Here's how the part is built. I have some questions about the finished solid (model axes, mm). Face numbers are marked on the shaded views. A direction names the side the tool comes from. Round coordinates to 2 decimals unless told otherwise and drop trailing zeros. Order: outer loops, then holes, each group sorted by start corner. A loop starts at its lowest first (then second) coordinate and runs counter-clockwise, first axis right, second up. Notation, with made-up numbers: (-29, 45.5) - (11, 45.5) arc R14 ccw to (11, 61.5) - close; hole circle Ø5 at (79.5, -1). An arc over 180 degrees is marked (long way). Answer as a JSON object with one key per item and string values.
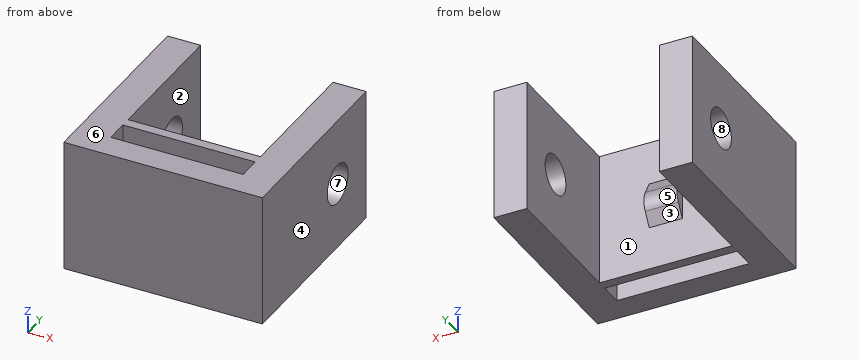
```python
from build123d import *

# Parameters (mm, degrees)
SKETCH1_W           = 10
SKETCH1_H           = 0.75
BOSS_EXTRUDE1_DEPTH = 10
BOSS_EXTRUDE2_DEPTH = 1.25
SKETCH2_5_R         = 1.5
CUT_EXTRUDE1_DEPTH  = 25
FILLET1_R           = 1.5


with BuildPart() as part:
    # Sketch1 → Boss-Extrude1 (new body)
    with BuildSketch(Plane.XY):
        Polygon((-4.83125, 6.8625), (-7.33125, 6.8625), (-7.33125, -8.1375), (7.66875, -8.1375), (7.66875, 6.8625), (5.16875, 6.8625), (5.16875, -3.6375), (5.16875, -4.3875), (5.16875, -6.1375), (-4.83125, -6.1375), (-4.83125, -4.3875), (-4.83125, -3.6375), align=None)
        with Locations((0.16875, -4.0125)):
            Rectangle(SKETCH1_W, SKETCH1_H)
    extrude(amount=BOSS_EXTRUDE1_DEPTH)

    # Sketch2 → Boss-Extrude2 (add, symmetric)
    with BuildSketch(Plane(origin=(0.16875, 0, 0), x_dir=(0, 0, -1), z_dir=(1, 0, 0))):
        Polygon((-5, -2.6375), (-6.732050808, -3.6375), (-3.267949192, -3.6375), align=None)
    extrude(amount=BOSS_EXTRUDE2_DEPTH, both=True)

    # Sketch2_5 → Cut-Extrude1 (cut, symmetric)
    with BuildSketch(Plane(origin=(0.16875, 0, 0), x_dir=(0, 0, -1), z_dir=(1, 0, 0))):
        with Locations(Location((-5, 2.730596766, 0), (0, 0, 90))):
            Circle(SKETCH2_5_R)
    extrude(amount=CUT_EXTRUDE1_DEPTH, both=True, mode=Mode.SUBTRACT)

    # Fillet1
    fillet1_edges = [part.edges().sort_by_distance(p)[0] for p in [
        (0.16875, -2.6375, 5),
    ]]
    fillet(fillet1_edges, radius=FILLET1_R)


solid = part.part
```
1. Imagine slicing it at A-A (z = 5). List the corners of the cut face in (x, y) for me.
Responses:
{"outline": "(-7.33, -8.14) - (7.67, -8.14) - (7.67, 1.23) - (5.17, 1.23) - (5.17, -3.64) - (1.42, -3.64) - (1.42, -2.87) - (-1.08, -2.87) - (-1.08, -3.64) - (-4.83, -3.64) - (-4.83, 1.23) - (-7.33, 1.23) - close; (-7.33, 4.23) - (-4.83, 4.23) - (-4.83, 6.86) - (-7.33, 6.86) - close; (5.17, 4.23) - (7.67, 4.23) - (7.67, 6.86) - (5.17, 6.86) - close; hole (-4.83, -6.14) - (5.17, -6.14) - (5.17, -4.39) - (-4.83, -4.39) - close"}
2. If I drill on L1, parallel to X at y = -4.5, z = 4; L2, parallel to Y at x = -2.75, z = 1.25; L3, parallel to Y at x = -5, z = 6, over which ranges is the centre line in solid material (lowest first)? Write a range as [from, to].
Responses:
{"L1": "[-7.33, -4.83], [5.17, 7.67]", "L2": "[-8.14, -6.14], [-4.39, -3.64]", "L3": "[-8.14, 1.61], [3.85, 6.86]"}
3. For P1, Ø3, axis at x = -4.5, y = -3.5, coming from the -Z side; P2, Ø4, axis at x = -2, z = 5.5, coming from the +Y side; P3, Ø1.8, axis at y = 2.73, z = 5, coming from the -X side, each with a flat end and sliding along its axis, tell me the tip position at first contact or that it passes through.
Responses:
{"P1": "z = 0", "P2": "y = -2.87", "P3": "through"}
4. Thinking about a two-plate mould opening in Y: for the marked faces 5, 6, 7 and 8, which applies, pulls with the +Y half, pulls with the -Y half, needs draft (parallel to the pull), parting line crosses it, or undercut?
Responses:
{"face 5": "pulls with the +Y half", "face 6": "needs draft", "face 7": "undercut", "face 8": "undercut"}
5. Imagine slicing it at C-C (y = 4.75). List the corners of the cut face in (x, z) for me.
Responses:
{"outline": "(-7.33, 0) - (-4.83, 0) - (-4.83, 10) - (-7.33, 10) - close; (5.17, 0) - (7.67, 0) - (7.67, 10) - (5.17, 10) - close"}
6. For the marked faces 1, 2, 3 and 4, which set-ups out of +Z, -Z, +X, -X, +Y, -Y let a thin tool reach every point of the face, with its end or its side?
Responses:
{"face 1": "+Y", "face 2": "+Z, -Z, +Y", "face 3": "-Z, +Y", "face 4": "+Z, -Z, +X, +Y, -Y"}
7. Imagine slicing it at B-B (x = -3). List the corners of the cut face in (y, z) for me, plus the area to 3 significant figures.
Responses:
{"outline": "(-8.14, 0) - (-6.14, 0) - (-6.14, 10) - (-8.14, 10) - close; (-4.39, 0) - (-3.64, 0) - (-3.64, 10) - (-4.39, 10) - close", "area": "27.5 mm2"}
8. Imagine slicing it at D-D (z = 9.5). List the corners of the cut face in (x, y) for me, plus the area to 4 significant figures.
Responses:
{"outline": "(-7.33, -8.14) - (7.67, -8.14) - (7.67, 6.86) - (5.17, 6.86) - (5.17, -3.64) - (-4.83, -3.64) - (-4.83, 6.86) - (-7.33, 6.86) - close; hole (-4.83, -6.14) - (5.17, -6.14) - (5.17, -4.39) - (-4.83, -4.39) - close", "area": "102.5 mm2"}
